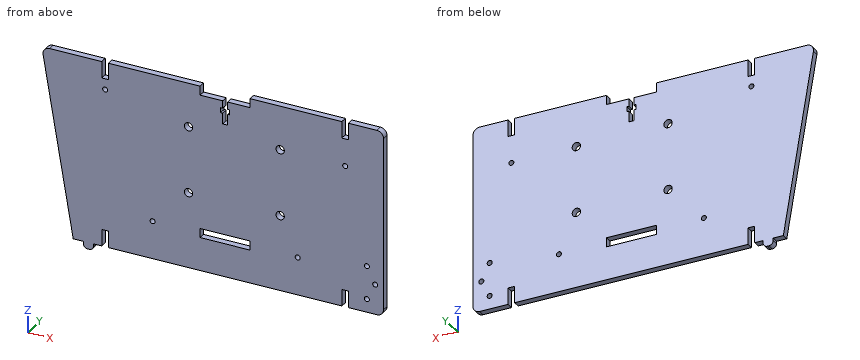
```python
from build123d import *

# Parameters (mm, degrees)
SKETCH1_R           = 1.5
SKETCH1_R_2         = 2.5
SKETCH1_W           = 30
SKETCH1_H           = 5.5
BOSS_EXTRUDE1_DEPTH = 4
FILLET1_R           = 4
FILLET3_R           = 4
FILLET4_R           = 4
FILLET5_R           = 2.5


with BuildPart() as part:
    # Sketch1 → Boss-Extrude1 (new body)
    with BuildSketch(Plane(origin=(0, 0, 0), x_dir=(1, 0, 0), z_dir=(0, 1, 0))):
        Polygon((158.5, 0), (180, 0), (180, 10), (184, 10), (184, 0), (205, 0), (205, 112), (184, 112), (184, 102), (180, 102), (180, 112), (40, 112), (40, 102), (36, 102), (36, 112), (31, 112), (31, 116), (25, 116), (25, 112), (18.8632, 112), (0, 0), (36, 0), (36, 10), (40, 10), (40, 0), (95, 0), (95, 5.5), (108.5, 5.5), (108.5, 10), (107.3, 10), (107.3, 13), (108.5, 13), (108.5, 19.5), (111.5, 19.5), (111.5, 13), (112.7, 13), (112.7, 10), (111.5, 10), (111.5, 5.5), (125, 5.5), (125, 0), (155.5, 0), align=None)
        with Locations(Location((153.5, 89.25, 0), (0, 0, 270))):
            Circle(SKETCH1_R, mode=Mode.SUBTRACT)
        with Locations(Location((66.5, 89.25, 0), (0, 0, 270))):
            Circle(SKETCH1_R, mode=Mode.SUBTRACT)
        with Locations(Location((88, 66.5, 0), (0, 0, 270))):
            Circle(SKETCH1_R_2, mode=Mode.SUBTRACT)
        with Locations(Location((88.007190659, 26.500000646, 0), (0, 0, 270))):
            Circle(SKETCH1_R_2, mode=Mode.SUBTRACT)
        with Locations(Location((143, 66.5, 0), (0, 0, 270))):
            Circle(SKETCH1_R_2, mode=Mode.SUBTRACT)
        with Locations(Location((143.007190659, 26.500000646, 0), (0, 0, 270))):
            Circle(SKETCH1_R_2, mode=Mode.SUBTRACT)
        with Locations(Location((195, 104, 0), (0, 0, 270))):
            Circle(SKETCH1_R, mode=Mode.SUBTRACT)
        with Locations(Location((195, 84, 0), (0, 0, 270))):
            Circle(SKETCH1_R, mode=Mode.SUBTRACT)
        with Locations(Location((200, 94, 0), (0, 0, 270))):
            Circle(SKETCH1_R, mode=Mode.SUBTRACT)
        with Locations(Location((182, 26.5, 0), (0, 0, 270))):
            Circle(SKETCH1_R, mode=Mode.SUBTRACT)
        with Locations(Location((38, 16.5, 0), (0, 0, 270))):
            Circle(SKETCH1_R, mode=Mode.SUBTRACT)
        with Locations((110, 89.25)):
            Rectangle(SKETCH1_W, SKETCH1_H, mode=Mode.SUBTRACT)
    extrude(amount=BOSS_EXTRUDE1_DEPTH)

    # Fillet1
    fillet1_edges = [part.edges().sort_by_distance(p)[0] for p in [
        (0, 2, 0),
    ]]
    fillet(fillet1_edges, radius=FILLET1_R)

    # Fillet3
    fillet3_edges = [part.edges().sort_by_distance(p)[0] for p in [
        (205, 2, -112),
    ]]
    fillet(fillet3_edges, radius=FILLET3_R)

    # Fillet4
    fillet4_edges = [part.edges().sort_by_distance(p)[0] for p in [
        (205, 2, 0),
    ]]
    fillet(fillet4_edges, radius=FILLET4_R)

    # Fillet5
    fillet5_edges = [part.edges().sort_by_distance(p)[0] for p in [
        (25, 2, -116),
        (31, 2, -116),
    ]]
    fillet(fillet5_edges, radius=FILLET5_R)


solid = part.part
```
The listing builds one solid part. Answer for the finished solid, in the listing's coordinates (mm). Coordinates: 2 decimals unless noted, no trailing zeros. Loops run counter-clockwise (first coordinate to the right, second up) from the corner with the lowest first, then second, coordinate; pieces in that order, holes last. Notation, with made-up numbers: (23.5, 21) - (67.5, 21) arc R25 ccw to (67.5, 40) - close; hole circle Ø1 at (49, 47). An arc over 180 degrees is marked (long way). Write item = value, one per line.
1) Section B-B (z = -66.5) is taken. Determine the outline of the cut face in (x, y), plus the area to 3 significant figures.
Responses:
outline = (11.2, 0) - (85.5, 0) - (85.5, 4) - (11.2, 4) - close; (90.5, 0) - (140.5, 0) - (140.5, 4) - (90.5, 4) - close; (145.5, 0) - (205, 0) - (205, 4) - (145.5, 4) - close
area = 735 mm^2
2) Section A-A (x = 118) is taken. Determine the outline of the cut face in (y, z).
Responses:
outline = (0, -112) - (4, -112) - (4, -92) - (0, -92) - close; (0, -86.5) - (4, -86.5) - (4, -5.5) - (0, -5.5) - close
3) Find the intervals of material crossed by line 1 along Z through (x, y) = (195, 1.3); line 2 along Z through (x, y) = (143, 2.05); line 3 along Z through (x, y) = (153.5, 0.9), in increasing order.
Responses:
line_1 = -112 to -105.5, -102.5 to -85.5, -82.5 to 0
line_2 = -112 to -69, -64 to -29, -24 to 0
line_3 = -112 to -90.75, -87.75 to 0
4) Section D-D (x = 160.5) is taken. Determine the outline of the cut face in (y, z).
Responses:
outline = (0, -112) - (4, -112) - (4, 0) - (0, 0) - close
5) Each of these flat-tipped pins is pushed along its axis until it touches: P1, Ø2, axis at x = 34.5, y = 2, coming from the -Z side; P2, Ø2, axis at y = 1, z = -100, coming from the -X side; P3, Ø0.8, axis at y = 2.5, z = -112.5, coming from the -X side. Where does it stop, or does it pass through?
Responses:
P1 = -112
P2 = 16.67
P3 = 25
6) Section C-C (z = -34) is taken. Determine the outline of the cut face in (x, y), plus the area to 3 significant figures.
Responses:
outline = (5.73, 0) - (205, 0) - (205, 4) - (5.73, 4) - close
area = 797 mm^2
